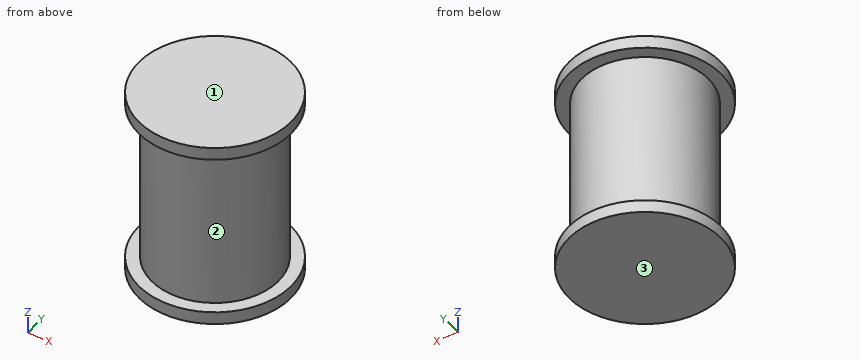
```python
from build123d import *

# Parameters (mm, degrees)
SKETCH_1_R        = 10
EXTRUDE_1_DEPTH   = 30
EXTRUDE_START     = -2
SKETCH_2_R        = 12
SKETCH_2_R_2      = 10
EXTRUDE_1_2_DEPTH = 2
SKETCH_3_R        = 12
SKETCH_3_R_2      = 10
EXTRUDE_2_DEPTH   = 2


with BuildPart() as part:
    # 草图1 → Extrude 1 (new body)
    with BuildSketch(Plane.XY):
        Circle(SKETCH_1_R)
    extrude(amount=EXTRUDE_1_DEPTH)

    # 草图2 → Extrude 1 2 (add)
    with BuildSketch(Plane.XY.offset(30).offset(EXTRUDE_START)):
        Circle(SKETCH_2_R)
        Circle(SKETCH_2_R_2, mode=Mode.SUBTRACT)
    extrude(amount=EXTRUDE_1_2_DEPTH)

    # 草图3 → 拉伸-薄壁2 (add)
    with BuildSketch(Plane(origin=(0, 0, 0), x_dir=(-1, 0, 0), z_dir=(0, 0, -1))):
        Circle(SKETCH_3_R)
        Circle(SKETCH_3_R_2, mode=Mode.SUBTRACT)
    extrude(amount=-EXTRUDE_2_DEPTH)


solid = part.part
```
Could you check a few things on this model? Use its own coordinates, in mm. Face numbers are marked on the shaded views. Round coordinates to 2 decimals unless told otherwise and drop trailing zeros. Write each loop counter-clockwise with the first axis right and the second up, starting at its lowest first coordinate (ties: lowest second). Pieces come first, ordered by that corner, then holes. Notation, with made-up numbers: M 0,57 L 14,57 A9 ccw 14,69 Z; hole C 61,13 d7. An arc over 180 degrees is marked long. Answer in a Markdown table with one row per item. Add a question column.
Q1. Will these pins go through, and if not, where does the flat tip stop? pin 1 Ø4 at (y, z) = (4, 19) entering from -X; pin 2 Ø12 at (x, z) = (-8.5, 16) entering from +Y; pin 3 Ø10 at (y, z) = (5.5, 8) entering from +X.
Q2. Imagine slicing it at C-C (z = 27.5). Please give me the cut outline in (x, y), then the cut area to 3 significant figures.
Q3. If I drill on line 1 (Z direction, x = 3, y = 10.5); line 2 (X direction, y = -9, z = 7.25); line 3 (Y direction, x = -4.5, z = 8.25), over which ranges is the centre line in solid material (lowest first)? Write a range as from..to.
Q4. If we mould it in two halves opening along Z, with no side actions, what happens to the marked faces 1, 2 and 3? For each: +Z half, -Z half, draft (parallel to the pull), parting line (faces both ways), or undercut.
Q5. Imagine slicing it at A-A (x = 0). Please give me the cut outline in (y, z), then the cut area to 3 significant figures.
Values:
| question | item | result |
|---|---|---|
| 1 | pin 1 | x = -9.8 |
| 1 | pin 2 | y = 9.68 |
| 1 | pin 3 | x = 9.99 |
| 2 | outline | C 0,0 d20 |
| 2 | area | 314 mm^2 |
| 3 | line 1 | 0..2, 28..30 |
| 3 | line 2 | -4.36..4.36 |
| 3 | line 3 | -8.93..8.93 |
| 4 | face 1 | +Z half |
| 4 | face 2 | undercut |
| 4 | face 3 | -Z half |
| 5 | outline | M -12,0 L 12,0 L 12,2 L 10,2 L 10,28 L 12,28 L 12,30 L -12,30 L -12,28 L -10,28 L -10,2 L -12,2 Z |
| 5 | area | 616 mm^2 |
